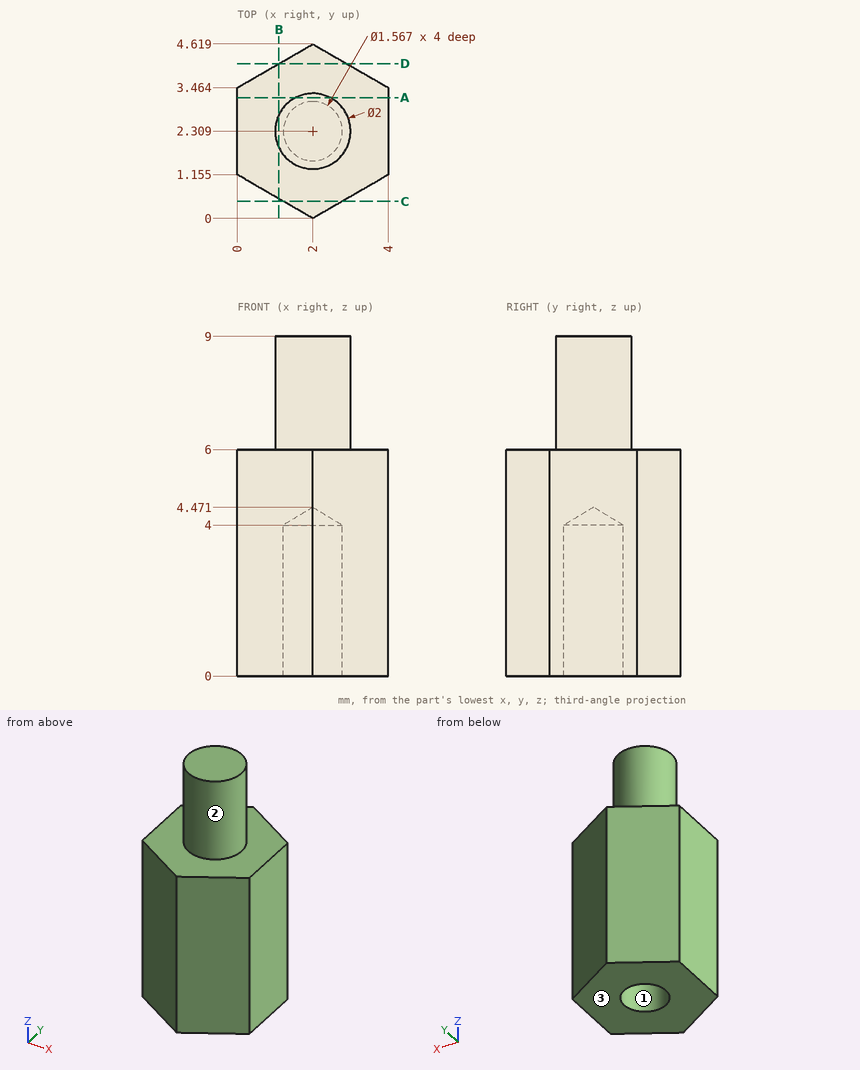
Verification items for this drawing (mm, ordinates from the low corner). A direction names the side the tool comes from. Coordinates: 2 decimals unless noted, no trailing zeros. Order: outer loops, then holes, each group sorted by start corner. A loop starts at its lowest first (then second) coordinate and runs counter-clockwise, first axis right, second up. Notation, with made-up numbers: (-11.5, 54) -> (37.5, 54) arc R35 cw to (37.5, 92) -> close; hole circle Ø7 at (42, -39.5). An arc over 180 degrees is marked (long way). Answer as CSV lines item,"result". Start each with the question number.
1) Cross-section at A-A, the plane y = 3.2. Record the boundary of the cut face in (x, z) (1 decimal), then the cut area to 3 significant figures.
2) Cross-section at B-B, the plane x = 1.1. Record the boundary of the cut face in (y, z) (1 decimal), then the cut area to 3 significant figures.
3) Set-up check for the marked faces 1, 2 and 3: record each of +Z, -Z, +X, -X, +Y, -Y from which the full face is reachable in a straight line by a thin tool's end or side.
4) Material ranges on L1, parallel to Z at x = 1.15, y = 1.65; L2, parallel to X at y = 1.85, z = 3.75 (1 decimal); L3, parallel to Y at x = 1.8, z = 1.75 (1 decimal), recorded low to high. Write a range as [from, to].
5) Cross-section at D-D, the plane y = 4.1. Record the boundary of the cut face in (x, z).
6) Cross-section at C-C, the plane y = 0.45. Record the boundary of the cut face in (x, z).
7) Gauge pin test, flat end, axial feed: pin 1 Ø1.5 at (x, z) = (1.5, 3) entering from -Y. Record the tip position at first contact, or that the pin passes through.
Conclusion:
1,outline,"(0, 0) -> (4, 0) -> (4, 6) -> (2.5, 6) -> (2.5, 9) -> (1.5, 9) -> (1.5, 6) -> (0, 6) -> close"
1,area,"26.7 mm²"
2,outline,"(0.5, 0) -> (4.1, 0) -> (4.1, 6) -> (2.7, 6) -> (2.7, 9) -> (1.9, 9) -> (1.9, 6) -> (0.5, 6) -> close"
2,area,"24.1 mm²"
3,face 1,"-Z"
3,face 2,"+Z"
3,face 3,"-Z, +X, -X, +Y, -Y"
4,L1,"z = [0, 6]"
4,L2,"x = [0, 1.4], [2.6, 4]"
4,L3,"y = [0.1, 1.6], [3.1, 4.5]"
5,outline,"(1.1, 0) -> (2.9, 0) -> (2.9, 6) -> (1.1, 6) -> close"
6,outline,"(1.22, 0) -> (2.78, 0) -> (2.78, 6) -> (1.22, 6) -> close"
7,pin 1,"stops at y = 0"
